Autodesk Inventor part; units mm, degrees
ref_plane "YZ Plane" through (0, 0, 0) normal (1, 0, 0) x (0, 1, 0)
ref_plane "XZ Plane" through (0, 0, 0) normal (0, 1, 0) x (-1, 0, 0)
ref_plane "XY Plane" through (0, 0, 0) normal (0, 0, 1) x (1, 0, 0)
sketch "Sketch1" plane through (0, 0, 0) normal (0, 1, 0) x (-1, 0, 0)
  line L0 (4.9142, 0) -> (0, 0)
  line L1 (0, 0) -> (0, 7.2679)
  circle A0 centre (12.7, 12.7) radius 1.5875
  circle A1 centre (25.4, 12.7) radius 1.5875
  circle A2 centre (38.1, 12.7) radius 1.5875
  circle A3 centre (50.8, 12.7) radius 1.5875
  circle A4 centre (12.7, 25.4) radius 1.5875
  circle A5 centre (12.7, 38.1) radius 1.5875
  circle A6 centre (12.7, 50.8) radius 1.5875
  circle A7 centre (12.7, 63.5) radius 1.5875
  circle A8 centre (12.7, 76.2) radius 1.5875
  line L2 (0, 7.2679) -> (0, 79.375)
  line L3 (3.175, 82.55) -> (22.225, 82.55)
  line L4 (25.4, 79.375) -> (25.4, 28.575)
  line L5 (28.575, 25.4) -> (53.975, 25.4)
  line L6 (57.15, 22.225) -> (57.15, 3.175)
  line L7 (53.975, 0) -> (4.9142, 0)
  line L8 (57.15, 22.225) -> (53.975, 25.4)
  line L9 (57.15, 3.175) -> (53.975, 0)
  line L10 (3.175, 82.55) -> (0, 79.375)
  line L11 (22.225, 82.55) -> (25.4, 79.375)
  arc A9 (25.4, 28.575) -> (28.575, 25.4) centre (28.575, 28.575) ccw
  point P0 (2.4571, 0)
  point P1 (0, 82.55)
  point P2 (25.4, 82.55)
  point P3 (25.4, 25.4)
  point P4 (57.15, 25.4)
  point P5 (57.15, 0)
  point P6 (57.15, 12.7)
  dimension "d0" = 3.175
  dimension "d1" = 12.7
  dimension "d2" = 12.7
  dimension "d5" = 12.7
  dimension "d12" = 12.7
  dimension "d17" = 25.4
  dimension "d18" = 6.35
  dimension "d19" = 12.7
  dimension "d20" = 6.35
  dimension "d21" = 3.175
  dimension "d22" = 3.175
  dimension "d23" = 3.175
  dimension "d24" = 3.175
  dimension "d25" = 3.175
  dimension "d26" = 3.175
  dimension "d27" = 3.175
  dimension "d28" = 3.175
  dimension "d29" = 3.175
extrude "Extrusion1" add sketch "Sketch1" along normal blind 3.175
properties part number "L-Bracket (4x6)"
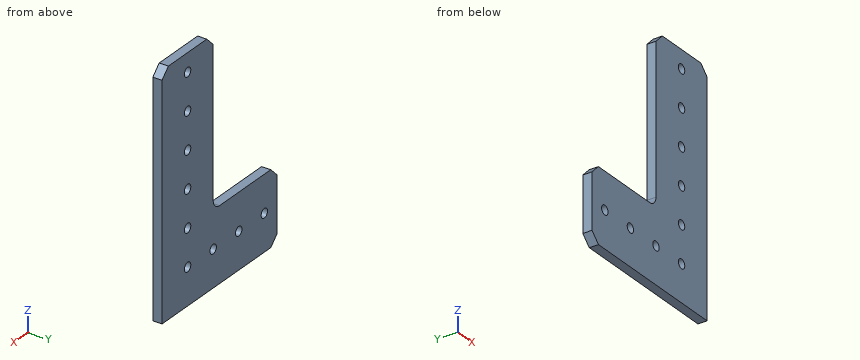
Model file for the job. Use its own axes, mm. Give positions to 0.01 mm unless a question says otherwise; leave off trailing zeros. Order: outer loops, then holes, each group sorted by start corner. A loop starts at its lowest first (then second) coordinate and runs counter-clockwise, first axis right, second up. Notation, with made-up numbers: M 26,61.5 L 47,61.5 A28 cw 47,83.5 Z; hole C 5.5,37 d10. An arc over 180 degrees is marked long. Put each result on its own line as item: value. Start each with the question number.
(1) Band-saw the part on A-A on x = -38.1. Give the cut face in (y, z) (1 decimal), then the cut area to 3 significant figures.
(2) Band-saw the part on B-B on y = 0.5. Count the separate pieces of the cut face and the enclosed holes in it, then the cut area to 3 significant figures.
(3) Pin check, flat tips, straight feed: pin 1 Ø4 at (x, z) = (-25.4, 12.7) entering from -Y; pin 2 Ø1 at (y, z) = (1.5, 65) entering from -X. Stop position of each tip, or through.
(4) Drill centre lines: L1, parallel to Z at x = -38, y = 2; L2, parallel to X at y = 0.3, z = 71; L3, parallel to Z at x = -51.5, y = 1.65. Where is each one in solid material? Low to high. Write a range as [from, to].
(5) Band-saw the part on C-C on z = 76.2. Give the cut face in (x, y) (1 decimal), then the cut area to 3 significant figures.
Results below:
1. outline: M 0,0 L 3.2,0 L 3.2,11.1 L 0,11.1 Z; M 0,14.3 L 3.2,14.3 L 3.2,25.4 L 0,25.4 Z
1. area: 70.6 mm2
2. separate pieces: 1
2. enclosed holes: 9
2. area: 2,810 mm2
3. pin 1: stops at y = 0
3. pin 2: stops at x = -25.4
4. L1: z = [0, 11.12], [14.28, 25.4]
4. L2: x = [-25.4, 0]
4. L3: z = [0, 11.28], [14.12, 25.4]
5. outline: M -25.4,0 L -14.3,0 L -14.3,3.2 L -25.4,3.2 Z; M -11.1,0 L 0,0 L 0,3.2 L -11.1,3.2 Z
5. area: 70.6 mm2
